from build123d import *

# Parameters (mm, degrees)
SKETCH1_R           = 10
SKETCH1_R_2         = 19
BOSS_EXTRUDE1_DEPTH = 128


with BuildPart() as part:
    # Sketch1 → Boss-Extrude1 (new body)
    with BuildSketch(Plane.XY):
        with BuildLine():
            ThreePointArc((20.542128414, 23.491399981), (-11.954310602, 39.999816289), (-44.350086912, 23.294726197))
            ThreePointArc((-44.350086912, 23.294726197), (-48.286212782, 20.194921951), (-53.269861719, 19.680027304))
            ThreePointArc((-53.269861719, 19.680027304), (-76.75292632, 1.788778062), (-56.833080109, -20))
            Line((-56.833080109, -20), (-46.474096261, -20))
            ThreePointArc((-46.474096261, -20), (-39.993245797, -28.407834632), (-31.528984999, -34.814814815))
            ThreePointArc((-31.528984999, -34.814814815), (-18.567319972, -53.9492851), (-25.962751008, -75.845410628))
            ThreePointArc((-25.962751008, -75.845410628), (-26.45371097, -103.646873387), (1.315633204, -105.070213608))
            ThreePointArc((1.315633204, -105.070213608), (35.455910615, -44.457444325), (20.542128414, 23.491399981))
        make_face()
        with Locations((-56.833080109, 0)):
            Circle(SKETCH1_R, mode=Mode.SUBTRACT)
        with Locations((-11.833080109, -90)):
            Circle(SKETCH1_R, mode=Mode.SUBTRACT)
        with Locations((-11.833080109, 0)):
            Circle(SKETCH1_R_2, mode=Mode.SUBTRACT)
    extrude(amount=BOSS_EXTRUDE1_DEPTH)


solid = part.part
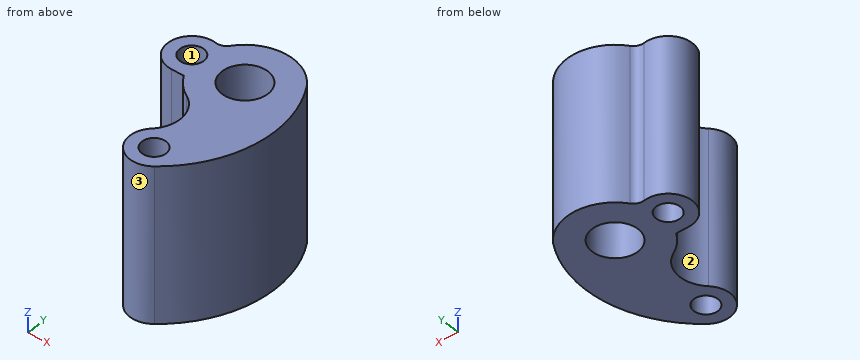
Input: part model. Units: mm. Frame: model coordinates. Face numbers are marked on the shaded views. Round coordinates to 2 decimals unless told otherwise and drop trailing zeros. Order: outer loops, then holes, each group sorted by start corner. A loop starts at its lowest first (then second) coordinate and runs counter-clockwise, first axis right, second up. Notation, with made-up numbers: (11.25, 87) - (49.25, 87) arc R19 ccw to (49.25, 109) - close; hole circle Ø3 at (79, 85.25). An arc over 180 degrees is marked (long way). Use a Markdown table: item, result.
1. Mould query, pull axis X, two halves, no side actions, for the marked faces 1, 2 and 3. Classes: +X half, -X half, draft (parallel to the pull), parting line (faces both ways), or undercut.
Evaluation:
| item | result |
|---|---|
| face 1 | undercut |
| face 2 | -X half |
| face 3 | parting line |
2. Section A-A on y = -90. Return the cut outline in (x, z), then the cut area to 3 significant figures.
Evaluation:
| item | result |
|---|---|
| outline | (-31.83, 0) - (-21.83, 0) - (-21.83, 128) - (-31.83, 128) - close; (-1.83, 0) - (15.92, 0) - (15.92, 128) - (-1.83, 128) - close |
| area | 3,550 mm^2 |
3. First-contact query: pin 1 (4 mm diameter, centred on y = -38.5, z = 16, fed in from +X); pin 2 (12 mm diameter, centred on x = 1.5, z = 97, fed in from -Y); pin 3 (3 mm diameter, centred on x = -19, y = -15.5, fed in from +Z); pin 4 (1.5 mm diameter, centred on x = -50.5, z = 89.5, fed in from -Y). Flat tips, straight axial feed; report the tip coordinate or a pass-through.
Evaluation:
| item | result |
|---|---|
| pin 1 | x = 36.31 |
| pin 2 | y = -108.61 |
| pin 3 | through |
| pin 4 | y = -20 |
4. Section D-D on x = -49. Return the cut outline in (y, z).
Evaluation:
| item | result |
|---|---|
| outline | (-20, 0) - (-6.22, 0) - (-6.22, 128) - (-20, 128) - close; (6.22, 0) - (19.94, 0) - (19.94, 128) - (6.22, 128) - close |
5. Section C-C on y = 3. Return the cut outline in (x, z), then the cut area to 3 significant figures.
Evaluation:
| item | result |
|---|---|
| outline | (-76.61, 0) - (-66.37, 0) - (-66.37, 128) - (-76.61, 128) - close; (-47.29, 0) - (-30.59, 0) - (-30.59, 128) - (-47.29, 128) - close; (6.93, 0) - (30.77, 0) - (30.77, 128) - (6.93, 128) - close |
| area | 6,500 mm^2 |
6. Section B-B on z = 114. Return the cut outline in (x, y).
Evaluation:
| item | result |
|---|---|
| outline | (-56.83, -20) - (-46.47, -20) arc R40 ccw to (-31.53, -34.81) arc R26 cw to (-25.96, -75.85) arc R20 ccw to (1.32, -105.07) arc R97.57 ccw to (20.54, 23.49) arc R40 ccw to (-44.35, 23.29) arc R9 cw to (-53.27, 19.68) arc R20 ccw (long way) to start; hole circle Ø20 at (-56.83, 0); hole circle Ø38 at (-11.83, 0); hole circle Ø20 at (-11.83, -90) |
7. Material intervals for probe 1 along Y at (x, z) = (-22.5, 84.5); probe 2 along X at (y, z) = (2, 110.5); probe 3 along Y at (x, z) = (-15, 121), sorted ascending.
Evaluation:
| item | result |
|---|---|
| probe 1 | -106.92 to -71.57, -43.32 to -15.72, 15.72 to 38.55 |
| probe 2 | -76.73 to -66.63, -47.04 to -30.73, 7.06 to 31.12 |
| probe 3 | -109.75 to -99.49, -80.51 to -18.73, 18.73 to 39.87 |
